Autodesk Inventor part; units mm, degrees
ref_plane "YZ Plane" through (0, 0, 0) normal (1, 0, 0) x (0, 1, 0)
ref_plane "XZ Plane" through (0, 0, 0) normal (0, 1, 0) x (-1, 0, 0)
ref_plane "XY Plane" through (0, 0, 0) normal (0, 0, 1) x (1, 0, 0)
sketch "Szkic1" plane through (0, 0, 0) normal (0, 0, 1) x (1, 0, 0)
  circle A0 centre (0, 0) radius 24
  circle A1 centre (0, 0) radius 8
  dimension "d0" = 48
  dimension "d1" = 16
extrude "Wyciągnięcie proste1" add sketch "Szkic1" along normal blind 12
sketch "Szkic2" plane through (0, 0, 0) normal (0, 0, -1) x (-1, 0, 0)
  circle A0 centre (0, 0) radius 8
  circle A1 centre (0, 0) radius 14
  dimension "d4" = 28
extrude "Wyciągnięcie proste2" add sketch "Szkic2" along normal blind 23
sketch "Szkic3" plane through (0, 0, 12) normal (0, 0, 1) x (1, 0, 0)
  circle A0 centre (0, 0) radius 19
  circle A1 centre (0, 19) radius 3
  circle A2 centre (16.4545, 9.5) radius 3
  circle A3 centre (16.4545, -9.5) radius 3
  circle A4 centre (0, -19) radius 3
  circle A5 centre (-16.4545, -9.5) radius 3
  circle A6 centre (-16.4545, 9.5) radius 3
  dimension "d7" = 38
  dimension "d8" = 6
  dimension "d11" = 360
extrude "Wyciągnięcie proste3" cut sketch "Szkic3" against normal up to next contours A2 A0 | A0 A2 | A3 A0 | A0 A3 | A1 A0 | A0 A1 | A4 A0 | A0 A4 | A6 A0 | A0 A6 | A5 A0 | A0 A5
properties part number "Nakrętka trapezowa kołnierzowa JFRM-2835TR16x4"
Geometry: final body of the model. Coordinates: model frame, mm. A direction names the side the tool comes from. Coordinates: 2 decimals unless noted, no trailing zeros. Order: outer loops, then holes, each group sorted by start corner. A loop starts at its lowest first (then second) coordinate and runs counter-clockwise, first axis right, second up. Notation, with made-up numbers: (27.5, -17.75) - (67.5, -17.75) arc R23 ccw to (67.5, -0.75) - close; hole circle Ø10 at (51, 74). An arc over 180 degrees is marked (long way). Write each question's results on one line, items separated by ' | '.
(1) Section query D-D, the plane z = 3.5. Return the cut outline in (x, y).
Values found:
outline: circle Ø48 at (0, 0); hole circle Ø6 at (-16.45, -9.5); hole circle Ø6 at (-16.45, 9.5); hole circle Ø16 at (0, 0); hole circle Ø6 at (0, -19); hole circle Ø6 at (0, 19); hole circle Ø6 at (16.45, -9.5); hole circle Ø6 at (16.45, 9.5)
(2) Section query B-B, the plane x = 0. Return the cut outline in (y, z), plus the area to 3 significant figures.
Values found:
outline: (-24, 0) - (-22, 0) - (-22, 12) - (-24, 12) - close; (-16, 0) - (-14, 0) - (-14, -23) - (-8, -23) - (-8, 12) - (-16, 12) - close; (8, -23) - (14, -23) - (14, 0) - (16, 0) - (16, 12) - (8, 12) - close; (22, 0) - (24, 0) - (24, 12) - (22, 12) - close | area: 516 mm²
(3) Line query: line 1 (Y direction, x = 0, z = 4.5); line 2 (Y direction, x = -2, z = -14.5); line 3 (Z direction, x = -13, y = 18.5). Output: solid intervals per line, ascending. Write a range as [from, to].
Values found:
line 1: y = [-24, -22], [-16, -8], [8, 16], [22, 24] | line 2: y = [-13.86, -7.75], [7.75, 13.86] | line 3: z = [0, 12]
(4) Section query A-A, the plane y = 0. Return the cut outline in (x, z).
Values found:
outline: (-24, 0) - (-14, 0) - (-14, -23) - (-8, -23) - (-8, 12) - (-24, 12) - close; (8, -23) - (14, -23) - (14, 0) - (24, 0) - (24, 12) - (8, 12) - close
(5) First-contact query: pin 1 Ø8 at (y, z) = (14.5, -17.5) entering from +X; pin 2 Ø8 at (x, z) = (19, -11) entering from +Y; pin 3 Ø5 at (x, z) = (3, 5.5) entering from -Y; pin 4 Ø10 at (x, z) = (-16.5, -16.5) entering from +Y. Flat tips, straight axial feed; report the tip coordinate or a pass-through.
Values found:
pin 1: stops at x = 9.26 | pin 2: passes through | pin 3: stops at y = -23.99 | pin 4: stops at y = 7.98
(6) Set-up query: faces 4 (the face through (10.3, -10.3, 0)), 5 (the face through (-6, 6, 12)). Return all of +Z, -Z, +X, -X, +Y, -Y with unobstructed straight access to the full face (end or side cutting, diameter ignored); none if empty.
Values found:
face 4: -Z | face 5: +Z, +X, -X, +Y, -Y
(7) Mould query, pull axis X, two halves, no side actions, for faces 1 (the face through (19.226, 8.351, 6.084)), 2 (the face through (-6, -6, -23)), 3 (the face through (-23.977, -1.055, 5.916)). Classes: +X half, -X half, draft (parallel to the pull), parting line (faces both ways), or undercut.
Values found:
face 1: undercut | face 2: draft | face 3: parting line
(8) Section query C-C, the plane x = 17.5. Return the cut outline in (y, z), plus the area to 3 significant figures.
Values found:
outline: (-16.42, 0) - (-12.31, 0) - (-12.31, 12) - (-16.42, 12) - close; (-6.69, 0) - (6.69, 0) - (6.69, 12) - (-6.69, 12) - close; (12.31, 0) - (16.42, 0) - (16.42, 12) - (12.31, 12) - close | area: 259 mm²
